from build123d import *


with BuildPart() as part:
    # Sketch 1 → Revolve 1 (revolve)
    with BuildSketch(Plane.XY, mode=Mode.PRIVATE) as revolve_1_sk:
        with BuildLine():
            Line((0.348765499, 102), (0, 102))
            Line((0, 102), (0, 100))
            Line((0, 100), (0.348765499, 100))
            ThreePointArc((0.348765499, 100), (15.715348338, 95.980731584), (27.146090618, 84.952380952))
            ThreePointArc((27.146090618, 84.952380952), (42.06705822, 53.253307392), (49.87846865, 19.1))
            Line((49.87846865, 19.1), (51.892138751, 19.1))
            ThreePointArc((51.892138751, 19.1), (43.995996323, 53.794523258), (28.853763297, 85.993464052))
            ThreePointArc((28.853763297, 85.993464052), (16.694591362, 97.724601734), (0.348765499, 102))
        make_face()
    revolve(revolve_1_sk.sketch.rotate(Axis((0, 0, 0), (1, 0, 0)), 90), axis=Axis((0, 0, 0), (1, 0, 0)))


solid = part.part
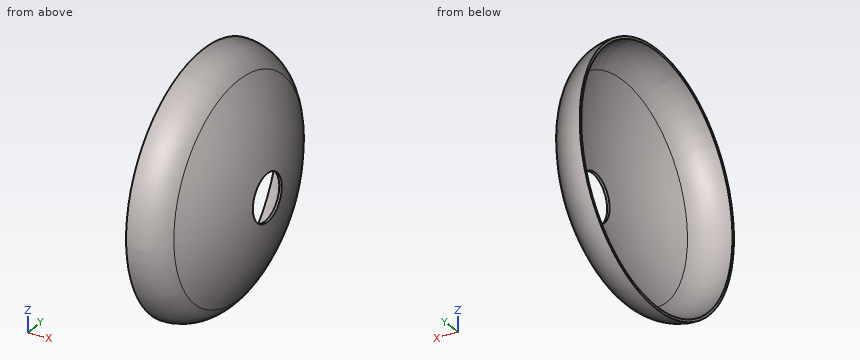
Work out the finished part from the listing and answer in its coordinate system (mm). Round coordinates to 2 decimals unless told otherwise and drop trailing zeros. Loops run counter-clockwise (first coordinate to the right, second up) from the corner with the lowest first, then second, coordinate; pieces in that order, holes last. Notation, with made-up numbers: (-27.75, 57.5) -> (-13.75, 57.5) arc R21 ccw to (-13.75, 92.5) -> close; hole circle Ø5 at (-24.75, 45.25). An arc over 180 degrees is marked (long way). Use one line per item in the form item = value.
(1) Find section C-C on x = 7. Give the vertices of the cut face in (y, z).
Answer list:
outline = circle Ø202.66 at (0, 0); hole circle Ø198.57 at (0, 0)
(2) Straight lines are drawn through the part: line 1 (Z direction, x = 10.5, y = -58); line 2 (Z direction, x = 11.5, y = -1.5); line 3 (Y direction, x = 14, z = 23.5). For each, find the intervals that lie inside material, in ascending order.
Answer list:
line_1 = -81.98 to -79.38, 79.38 to 81.98
line_2 = -100.07 to -97.94, 97.94 to 100.07
line_3 = -96.25 to -93.98, 93.98 to 96.25
(3) Find section A-A on y = 0. Give the vertices of the cut face in (x, z).
Answer list:
outline = (0, -102) -> (0.35, -102) arc R33.38 ccw to (28.85, -85.99) arc R165.2 ccw to (51.89, -19.1) -> (49.88, -19.1) arc R163.2 cw to (27.15, -84.95) arc R31.38 cw to (0.35, -100) -> (0, -100) -> close; (0, 100) -> (0.35, 100) arc R31.38 cw to (27.15, 84.95) arc R163.2 cw to (49.88, 19.1) -> (51.89, 19.1) arc R165.2 ccw to (28.85, 85.99) arc R33.38 ccw to (0.35, 102) -> (0, 102) -> close
(4) Find section D-D on x = 33. Give the vertices of the cut face in (y, z), then the cut area to 3 significant figures.
Answer list:
outline = circle Ø157.58 at (0, 0); hole circle Ø149.01 at (0, 0)
area = 2,060 mm2
(5) Flat-ended cylindrical pins translate along their axes: P1, Ø5, axis at x = 34.5, z = -16.5, coming from the +Y side; P2, Ø2, axis at y = -5.5, z = -75.5, coming from the +X side; P3, Ø6, axis at x = 13, y = -68, coming from the -Z side. Find the tip coordinate at first contact, or state that the pin passes through.
Answer list:
P1 = 78.93
P2 = 35.15
P3 = -75.76
